Autodesk Inventor part; units mm, degrees
ref_plane "YZ Plane" through (0, 0, 0) normal (1, 0, 0) x (0, 1, 0)
ref_plane "XZ Plane" through (0, 0, 0) normal (0, 1, 0) x (-1, 0, 0)
ref_plane "XY Plane" through (0, 0, 0) normal (0, 0, 1) x (1, 0, 0)
sketch "Sketch2" plane through (0, 0, 0) normal (0, 1, 0) x (-1, 0, 0)
  line L0 (-27.2, 0) -> (20.4, 0)
  line L1 (0, 8.6664) -> (0, 28.1819)
  line L2 (-17, 11) -> (-17, 24)
  line L3 (-17, 24) -> (17.8478, 24)
  arc A0 (-17, 11) -> (17.8478, 24) centre (0, 18.6364) ccw
  dimension "d1" = 24
  dimension "d2" = 18.6364
  dimension "d3" = 17
  dimension "d4" = 18.6364
extrude "Extrusion1" add sketch "Sketch2" along normal blind 10
The model under review builds one solid part; all positions refer to its coordinate system, in mm. Coordinates: 2 decimals unless noted, no trailing zeros. Loops run counter-clockwise (first coordinate to the right, second up) from the corner with the lowest first, then second, coordinate; pieces in that order, holes last. Notation, with made-up numbers: M 31,-38.75 L 49,-38.75 A27 ccw 49,-6.75 Z; hole C 69.25,76.25 d3. An arc over 180 degrees is marked long. Put each result on its own line as item: value. Start each with the question number.
Q1. Add section B-B (x = 14.5). Write out the cut boundary in (y, z), and give its area (3 significant figures).
Q2. Add section C-C (z = 4.25). Write out the cut boundary in (x, y).
Q3. Add section A-A (y = 2.75). Write out the cut boundary in (x, z), and give its area (3 significant figures).
Q4. Wall thickness on line 1 (Z direction, x = 7, y = 5.75); line 2 (X direction, y = 9.5, z = 5); line 3 (Z direction, x = 14, y = 4.75): over which ranges is each line inside the solid? List them lowest first.
Answers:
1. outline: M 0,6.93 L 10,6.93 L 10,24 L 0,24 Z
1. area: 171 mm^2
2. outline: M -11.85,0 L 11.85,0 L 11.85,10 L -11.85,10 Z
3. outline: M -17.85,24 A18.64 ccw 17,11 L 17,24 Z
3. area: 727 mm^2
4. line 1: z = 1.36 to 24
4. line 2: x = -12.7 to 12.7
4. line 3: z = 6.34 to 24
